Could you check a few things on this model? Use its own coordinates, in mm. A direction names the side the tool comes from. Coordinates: 2 decimals unless noted, no trailing zeros.
from build123d import *

# Parameters (mm, degrees)
SKETCH1_W           = 70
SKETCH1_H           = 70
BOSS_EXTRUDE1_DEPTH = 50
SKETCH8_R           = 2.5
CUT_EXTRUDE1_DEPTH  = 50


with BuildPart() as part:
    # Sketch1 → Boss-Extrude1 (new body)
    with BuildSketch(Plane.XY):
        with Locations((-35, -35)):
            Rectangle(SKETCH1_W, SKETCH1_H)
    extrude(amount=BOSS_EXTRUDE1_DEPTH)

    # Cut-Loft1: read off the stored shape, not the designer's step
    # Cut-Loft1: loft between two sections, ruled curve by curve
    cut_loft1_from = [
        Edge.make_bspline([(-19.308746069, -13.027641226, 10), (-63.253463616, 18.354866636, 10), (-94.635971478, -25.589850912, 10), (-50.691253931, -56.972358774, 10), (-6.746536384, -88.354866636, 10), (24.635971478, -44.410149088, 10), (-19.308746069, -13.027641226, 10)], [0, 0, 0, 0, 0.5, 0.5, 0.5, 1, 1, 1, 1], 3, [1, 0.333333333, 0.333333333, 1, 0.333333333, 0.333333333, 1]),
    ]
    cut_loft1_to = [
        Edge.make_bspline([(-22.079724584, -6.336756909, 50), (-79.406210767, 19.503793923, 50), (-105.246761599, -37.82269226, 50), (-47.920275416, -63.663243091, 50), (9.406210767, -89.503793923, 50), (35.246761599, -32.17730774, 50), (-22.079724584, -6.336756909, 50)], [0, 0, 0, 0, 0.5, 0.5, 0.5, 1, 1, 1, 1], 3, [1, 0.333333333, 0.333333333, 1, 0.333333333, 0.333333333, 1]),
    ]
    cut_loft1 = Solid(Shell([*[Face.make_surface_from_curves(cut_loft1_from[k], cut_loft1_to[k]) for k in range(1)], Face(Wire(cut_loft1_from)), Face(Wire(cut_loft1_to))]))
    add(cut_loft1, mode=Mode.SUBTRACT)

    # Sketch8 → Cut-Extrude1 (cut)
    with BuildSketch(Plane.XY.offset(10)):
        with Locations((-27.5, -35)):
            Circle(SKETCH8_R)
        with Locations(Location((-42.5, -35, 0), (0, 0, 180))):
            Circle(SKETCH8_R)
    extrude(amount=-CUT_EXTRUDE1_DEPTH, mode=Mode.SUBTRACT)


solid = part.part
(1) Which directions (+Z, -Z, +X, -X, +Y, -Y) give clear straight access to the entire face, cutting with the end or side of a thin tool? Please do faces 5 (the face through (-35, -39, 10)), 6 (the face through (-29, -33, 5)).
Answers:
face 5: +Z
face 6: +Z, -Z
(2) For pin 1 (3 mm diameter, centred on x = -27.5, y = -35, fed in from +Z); pin 2 (1 mm diameter, centred on x = -45, y = -12.5, fed in from +Z), each with a flat end and sliding along its axis, tell me the tip position at first contact or that it passes through.
Answers:
pin 1: passes through
pin 2: stops at z = 10
(3) We'd pull the mould along Y, two halves only. Please class faces 1 (the face through (0, -35, 25)), 2 (the face through (-35, -70, 25)), 3 (the face through (-35, 0, 25)), 4 (the face through (-44.81, -34.04, 5.07)): +Y half, -Y half, draft (parallel to the pull), parting line (faces both ways), or undercut.
Answers:
face 1: draft
face 2: -Y half
face 3: +Y half
face 4: undercut
(4) Imagine slicing it at A-A, the plane y = -35. State how many separate pieces and enclosed holes the cut face has, and give its area (3 significant figures).
Answers:
separate pieces: 3
enclosed holes: 0
area: 1,070 mm2
(5) I need wall thicknesses on probe 1 along Y at (x, z) = (-42.5, 6.25); probe 2 along Z at (x, y) = (-47, -41.5); probe 3 along Y at (x, z) = (-48.5, 33). Which ranges of each line are inside material? Lowest first, please.
Answers:
probe 1: y = -70 to -37.5, -32.5 to 0
probe 2: z = 0 to 10
probe 3: y = -70 to -61.14, -8.86 to 0
